The listing builds one solid part. Answer for the finished solid, in the listing's coordinates (mm). A direction names the side the tool comes from. Round coordinates to 2 decimals unless told otherwise and drop trailing zeros. Write each loop counter-clockwise with the first axis right and the second up, starting at its lowest first coordinate (ties: lowest second). Pieces come first, ordered by that corner, then holes.
from build123d import *

# Parameters (mm, degrees)
EXTRUDE_1_DEPTH     = 20
SKETCH_2_R          = 2.2
CUT_EXTRUDE_1_DEPTH = 20


with BuildPart() as part:
    # 草图1 → 凸台-拉伸1 (new body)
    with BuildSketch(Plane.XY):
        with BuildLine():
            Line((-46, 30), (46, 30))
            ThreePointArc((46, 30), (48.828427125, 28.828427125), (50, 26))
            Line((50, 26), (50, 0))
            Line((50, 0), (90, 0))
            Line((90, 0), (90, 6))
            ThreePointArc((90, 6), (88.828427125, 8.828427125), (86, 10))
            Line((86, 10), (64, 10))
            ThreePointArc((64, 10), (61.171572875, 11.171572875), (60, 14))
            Line((60, 14), (60, 36))
            ThreePointArc((60, 36), (58.828427125, 38.828427125), (56, 40))
            Line((56, 40), (-56, 40))
            ThreePointArc((-56, 40), (-58.828427125, 38.828427125), (-60, 36))
            Line((-60, 36), (-60, 14))
            ThreePointArc((-60, 14), (-61.171572875, 11.171572875), (-64, 10))
            Line((-64, 10), (-86, 10))
            ThreePointArc((-86, 10), (-88.828427125, 8.828427125), (-90, 6))
            Line((-90, 6), (-90, 0))
            Line((-90, 0), (-50, 0))
            Line((-50, 0), (-50, 26))
            ThreePointArc((-50, 26), (-48.828427125, 28.828427125), (-46, 30))
        make_face()
    extrude(amount=EXTRUDE_1_DEPTH)

    # 草图2 → 切除-拉伸1 (cut)
    with BuildSketch(Plane(origin=(0, 10, 0), x_dir=(1, 0, 0), z_dir=(0, 1, 0))):
        with Locations(Location((-80.5, -10, 0), (0, 0, 270))):
            Circle(SKETCH_2_R)
        with Locations(Location((-69.5, -10, 0), (0, 0, 270))):
            Circle(SKETCH_2_R)
        with Locations(Location((69.5, -10, 0), (0, 0, 270))):
            Circle(SKETCH_2_R)
        with Locations(Location((80.5, -10, 0), (0, 0, 270))):
            Circle(SKETCH_2_R)
    extrude(amount=-CUT_EXTRUDE_1_DEPTH, mode=Mode.SUBTRACT)


solid = part.part
1. For a pull along Z with two mould halves and no side action, classify faces 4 (the face through (82.68, 5.07, 9.71)), 5 (the face through (-60, 25, 10)), 6 (the face through (6.2, 30.5, 0)) as released by +Z, released by -Z, zero draft, split by the parting line, or undercut.
Geometry says:
face 4: undercut
face 5: zero draft
face 6: released by -Z
2. Section B-B on z = 10 is taken. Give the number of separate pieces and of enclosed holes in the cut face, plus the area to 3 significant figures.
Geometry says:
separate pieces: 5
enclosed holes: 0
area: 2,220 mm2
3. Section C-C on z = 16.75 is taken. Determine the outline of the cut face in (x, y), plus the area to 3 significant figures.
Geometry says:
outline: (-90, 0) - (-50, 0) - (-50, 26) arc R4 cw to (-46, 30) - (46, 30) arc R4 cw to (50, 26) - (50, 0) - (90, 0) - (90, 6) arc R4 ccw to (86, 10) - (64, 10) arc R4 cw to (60, 14) - (60, 36) arc R4 ccw to (56, 40) - (-56, 40) arc R4 ccw to (-60, 36) - (-60, 14) arc R4 cw to (-64, 10) - (-86, 10) arc R4 ccw to (-90, 6) - close
area: 2,400 mm2
4. Section D-D on x = -38.5 is taken. Determine the outline of the cut face in (y, z), plus the area to 3 significant figures.
Geometry says:
outline: (30, 0) - (40, 0) - (40, 20) - (30, 20) - close
area: 200 mm2
5. Straight lines are drawn through the part: line 1 along X through (y, z) = (5, 10); line 2 along X through (y, z) = (6.5, 4.5); line 3 along X through (y, z) = (19.5, 11.5). For each, find the intervals that lie inside material, in ascending order.
Geometry says:
line 1: x = -90 to -82.7, -78.3 to -71.7, -67.3 to -50, 50 to 67.3, 71.7 to 78.3, 82.7 to 90
line 2: x = -89.97 to -50, 50 to 89.97
line 3: x = -60 to -50, 50 to 60
6. Given pin 1 (1 mm diameter, centred on y = 27.5, z = 3.5, fed in from -X); pin 2 (6 mm diameter, centred on x = -26, z = 17, fed in from -Y); pin 3 (6 mm diameter, centred on y = 15.5, z = 7, fed in from +X); pin 4 (3.5 mm diameter, centred on x = 80.5, z = 10, fed in from +Y), each flat-ended and moving along its own axis, determine where each tip first touches the part or whether it passes through.
Geometry says:
pin 1: stops at x = -60
pin 2: stops at y = 30
pin 3: stops at x = 60.29
pin 4: passes through
7. A tool of negligible diameter and unlimited length cuts with its end or side. For faces 1 (the face through (50, 13, 10)), 2 (the face through (-75, 10, 10)), 3 (the face through (75, 10, 10)), from which of +Z, -Z, +X, -X, +Y, -Y can it reach the whole face along a straight path? Write none if from no direction.
Geometry says:
face 1: +Z, -Z, -Y
face 2: +Z, -Z, -X, +Y
face 3: +Z, -Z, +X, +Y
8. Section A-A on x = 69.5 is taken. Determine the outline of the cut face in (y, z), plus the area to 3 significant figures.
Geometry says:
outline: (0, 0) - (10, 0) - (10, 7.8) - (0, 7.8) - close; (0, 12.2) - (10, 12.2) - (10, 20) - (0, 20) - close
area: 156 mm2
